Input: part model. Units: mm. Frame: model coordinates. A direction names the side the tool comes from. Coordinates: 2 decimals unless noted, no trailing zeros. Order: outer loops, then holes, each group sorted by start corner. A loop starts at its lowest first (then second) coordinate and runs counter-clockwise, first axis right, second up.
from build123d import *

# Parameters (mm, degrees)
F0_W     = 7
F0_H     = 7
F1_DEPTH = 13.5
F2_W     = 4.3
F2_H     = 20.3
F3_DEPTH = 4.3
F4_DEPTH = 0.5
F5_R     = 0.75


with BuildPart() as f1:
    # F0 (on Front) → F1 (new body, symmetric)
    with BuildSketch(Plane.XZ):
        Rectangle(F0_W, F0_H)
    extrude(amount=F1_DEPTH, both=True)

    # F2 (on face) → F3 (cut)
    with BuildSketch(Plane.XY.offset(3.5)):
        Rectangle(F2_W, F2_H)
    extrude(amount=-F3_DEPTH, mode=Mode.SUBTRACT)

    # F4 (cut): a face of the model
    f4_faces = [f1.faces().sort_by_distance(p)[0] for p in [
        (0, 0, -3.5),
    ]]
    extrude(f4_faces, amount=-F4_DEPTH, mode=Mode.SUBTRACT)

    # F5
    f5_edges = [f1.edges().sort_by_distance(p)[0] for p in [
        (-3.5, 13.5, 0.25),
        (3.5, 13.5, 0.25),
        (3.5, -13.5, 0.25),
        (-3.5, -13.5, 0.25),
    ]]
    fillet(f5_edges, radius=F5_R)


solid = f1.part
Item 1: Cut plane B-B on y = -7.75. Return loops of the section in (x, z), then the cut area to 3 significant figures.
Response values:
outline: (-3.5, -3) - (3.5, -3) - (3.5, 3.5) - (2.15, 3.5) - (2.15, -0.8) - (-2.15, -0.8) - (-2.15, 3.5) - (-3.5, 3.5) - close
area: 27.0 mm2
Item 2: Access query for faces 1 (the face through (0, 13.5, 0)), 2 (the face through (0, -10.15, 1)). Directions: +Z, -Z, +X, -X, +Y, -Y. A direction counts if a zero-diameter tool reaches every point of the face in a straight line with its end or side. Return the directions, or none.
Response values:
face 1: +Z, -Z, +X, -X, +Y
face 2: +Z
Item 3: Pin query (flat end, axial travel): pin 1 Ø1.3 at (x, y) = (-0.5, 3) entering from +Z. Return the tip coordinate at first contact, or that it passes through.
Response values:
pin 1: stops at z = -0.8
Item 4: Cut plane C-C on x = 1.5. Return loops of the section in (y, z).
Response values:
outline: (-13.5, -3) - (13.5, -3) - (13.5, 3.5) - (10.15, 3.5) - (10.15, -0.8) - (-10.15, -0.8) - (-10.15, 3.5) - (-13.5, 3.5) - close
Item 5: Draft query along X for faces 3 (the face through (-3.5, 0, 0)), 4 (the face through (2.15, 0, 1)), 5 (the face through (3.5, 0, 0)). Return one class per face: pulls with the +X half, pulls with the -X half, needs draft (parallel to the pull), parting line crosses it, or undercut.
Response values:
face 3: pulls with the -X half
face 4: undercut
face 5: pulls with the +X half
Item 6: Cut plane A-A on z = 2.25. Return loops of the section in (x, y).
Response values:
outline: (-3.5, -12.75) arc R0.75 ccw to (-2.75, -13.5) - (2.75, -13.5) arc R0.75 ccw to (3.5, -12.75) - (3.5, 12.75) arc R0.75 ccw to (2.75, 13.5) - (-2.75, 13.5) arc R0.75 ccw to (-3.5, 12.75) - close; hole (-2.15, -10.15) - (2.15, -10.15) - (2.15, 10.15) - (-2.15, 10.15) - close
Item 7: Ray query, probe 1 along X at (y, z) = (-4.5, 0); probe 2 along Y at (x, z) = (1.75, 2); probe 3 along Z at (x, y) = (-0.5, -7.5). Return the intervals inside material, ascending.
Response values:
probe 1: x = -3.5 to -2.15, 2.15 to 3.5
probe 2: y = -13.5 to -10.15, 10.15 to 13.5
probe 3: z = -3 to -0.8
